Source: CAD feature listing. Evaluate the final solid. Frame: model axes, mm. A direction names the side the tool comes from. Round coordinates to 2 decimals unless told otherwise and drop trailing zeros. Order: outer loops, then holes, each group sorted by start corner. A loop starts at its lowest first (then second) coordinate and runs counter-clockwise, first axis right, second up. Notation, with made-up numbers: (-20.5, 6) - (-0.5, 6) arc R15 cw to (-0.5, 26) - close; hole circle Ø5 at (61.5, 60.5). An arc over 180 degrees is marked (long way). Use one line per item in the form item = value. Start each with the question number.
Q1. Cut plane B-B, the plane x = -17. Return the cut outline in (y, z) (3 decimals), and give its area (3 significant figures).
Q2. Set-up query: faces 5 (the cylindrical face through (-16.41, 1.97, 22.26)), 6 (the cylindrical face through (16.41, 1.97, 0.6)), 7 (the flat face through (-14, -1, 19.685)), 8 (the cylindrical face through (16.37, 1.97, 22.26)), 9 (the flat face through (-10.643, -1, 21)). Return all of +Z, -Z, +X, -X, +Y, -Y with unobstructed straight access to the full face (end or side cutting, diameter ignored); none if empty.
Q3. Pin query (flat end, axial travel): pin 1 Ø3.5 at (x, z) = (20.17, 11.43) entering from +Y; pin 2 Ø1.3 at (y, z) = (-1.5, 2) entering from +X; pin 3 Ø3 at (y, z) = (-1, 2) entering from -X. Return the tip coordinate at first contact, or that it passes through.
Q4. Cut plane C-C, the plane x = 0. Return the cut outline in (y, z), and give its area (3 significant figures).
Q5. Ray query, line 1 (X direction, y = 1.05, z = 11.43); line 2 (Y direction, x = 25.5, z = 11.75); line 3 (X direction, y = 3.75, z = 8.5). Return the intervals inside material, ascending. Write a range as [from, to].
Q6. Draft query along X for faces 1 (the cylindrical face through (-13.94, 2.95, 11.3)), 2 (the flat face through (10.643, -1, 2)), 3 (the cylindrical face through (-18.657, 1.288, 11.232)), 4 (the cylindrical face through (0.248, 13.815, 11.298)). Return one class per face: released by +X, released by -X, zero draft, split by the parting line, or undercut.
Q7. Cut plane A-A, the plane z = 11.43. Return the cut outline in (x, y), and give its area (3 significant figures).
from build123d import *

# Parameters (mm, degrees)
BOSS_EXTRUDE1_DEPTH      = 22.86
BOSS_EXTRUDE8_DEPTH      = 2.54
BOSS_EXTRUDE8_DEPTH_BACK = 2.54
SKETCH9_W                = 3.175
SKETCH9_H                = 22.86
BOSS_EXTRUDE9_DEPTH      = 2.54
BOSS_EXTRUDE9_DEPTH_BACK = 2.54
SKETCH10_W               = 3.175
SKETCH10_H               = 22.86
BOSS_EXTRUDE10_DEPTH     = 3.81
BOSS_EXTRUDE11_DEPTH     = 3.81
REVOLVE1_ANGLE           = 180
REVOLVE2_ANGLE           = 180
SKETCH22_W               = 16.51
SKETCH22_H               = 2.54
CUT_EXTRUDE1_DEPTH       = 3.81
SKETCH23_W               = 16.51
SKETCH23_H               = 2.54
CUT_EXTRUDE2_DEPTH       = 3.81
SKETCH24_R               = 1.524
CUT_EXTRUDE3_DEPTH       = 3.81
FILLET1_R                = 2


with BuildPart() as part:
    # Sketch1 → Boss-Extrude1 (new body)
    with BuildSketch(Plane.XY):
        with BuildLine():
            Line((-13.8176, 0), (-10.6426, 0))
            ThreePointArc((-10.6426, 0), (0, 10.6426), (10.6426, 0))
            Line((10.6426, 0), (13.8176, 0))
            ThreePointArc((13.8176, 0), (0, 13.8176), (-13.8176, 0))
        make_face()
    extrude(amount=BOSS_EXTRUDE1_DEPTH)

    # Sketch9 → Boss-Extrude8 (add, two sides: drawn at the far end of the back side and taken through both)
    with BuildSketch(Plane.XZ.offset(-BOSS_EXTRUDE8_DEPTH_BACK)):
        with Locations((-12.2301, 11.43)):
            Rectangle(SKETCH9_W, SKETCH9_H)
    extrude(amount=BOSS_EXTRUDE8_DEPTH + BOSS_EXTRUDE8_DEPTH_BACK)

    # Sketch10 → Boss-Extrude9 (add, two sides: drawn at the far end of the back side and taken through both)
    with BuildSketch(Plane.XZ.offset(-BOSS_EXTRUDE9_DEPTH_BACK)):
        with Locations((12.2301, 11.43)):
            Rectangle(SKETCH10_W, SKETCH10_H)
    extrude(amount=BOSS_EXTRUDE9_DEPTH + BOSS_EXTRUDE9_DEPTH_BACK)

    # Sketch11 → Boss-Extrude10 (add)
    with BuildSketch(Plane.ZY.offset(13.8176)):
        Polygon((22.86, 2.54), (0, 2.54), (0, 0), (0, -2.54), (3.175, -2.54), (3.175, 0), (19.685, 0), (19.685, -2.54), (22.86, -2.54), align=None)
    extrude(amount=BOSS_EXTRUDE10_DEPTH)

    # Sketch19 → Boss-Extrude11 (add)
    with BuildSketch(Plane(origin=(13.8176, 0, 0), x_dir=(0, 0, -1), z_dir=(1, 0, 0))):
        Polygon((-19.685, -2.54), (-19.685, 0), (-3.175, 0), (-3.175, -2.54), (0, -2.54), (0, 2.54), (-22.86, 2.54), (-22.86, -2.54), align=None)
    extrude(amount=BOSS_EXTRUDE11_DEPTH)

    # Sketch20 → Revolve1 (revolve)
    with BuildSketch(Plane.ZY.offset(17.6276)):
        Polygon((11.43, 2.54), (11.43, 0), (19.685, 0), (19.685, -2.54), (22.86, -2.54), (22.86, 2.54), align=None)
    revolve(axis=Axis((-17.6276, 2.54, 11.43), (0, -1, 0)), revolution_arc=REVOLVE1_ANGLE)

    # Sketch21 → Revolve2 (revolve)
    with BuildSketch(Plane(origin=(17.6276, 0, 0), x_dir=(0, 0, -1), z_dir=(1, 0, 0))):
        Polygon((-11.43, 2.54), (-11.43, 0), (-3.175, 0), (-3.175, -2.54), (0, -2.54), (0, 2.54), align=None)
    revolve(axis=Axis((17.6276, 2.54, 11.43), (0, -1, 0)), revolution_arc=REVOLVE2_ANGLE)

    # Sketch22 → Cut-Extrude1 (cut)
    with BuildSketch(Plane.ZY.offset(13.8176)):
        with Locations((11.43, -1.27)):
            Rectangle(SKETCH22_W, SKETCH22_H)
    extrude(amount=-CUT_EXTRUDE1_DEPTH, mode=Mode.SUBTRACT)

    # Sketch23 → Cut-Extrude2 (cut)
    with BuildSketch(Plane(origin=(13.8176, 0, 0), x_dir=(0, 0, -1), z_dir=(1, 0, 0))):
        with Locations((-11.43, -1.27)):
            Rectangle(SKETCH23_W, SKETCH23_H)
    extrude(amount=-CUT_EXTRUDE2_DEPTH, mode=Mode.SUBTRACT)

    # Sketch24 → Cut-Extrude3 (cut)
    with BuildSketch(Plane(origin=(0, 2.54, 0), x_dir=(1, 0, 0), z_dir=(0, 1, 0))):
        with Locations(Location((-20.1676, -11.43, 0), (0, 0, 270))):
            Circle(SKETCH24_R)
        with Locations(Location((20.1676, -11.43, 0), (0, 0, 270))):
            Circle(SKETCH24_R)
    extrude(amount=-CUT_EXTRUDE3_DEPTH, mode=Mode.SUBTRACT)

    # Fillet1
    fillet1_edges = [part.edges().sort_by_distance(p)[0] for p in [
        (-29.0576, 2.54, 11.43),
        (29.0576, 2.54, 11.43),
        (-15.604868947, 2.54, 0),
        (-15.604868947, 2.54, 22.86),
        (-13.582137894, 2.54, 11.43),
        (0, 13.8176, 0),
        (0, 13.8176, 22.86),
        (15.604868947, 2.54, 0),
        (15.604868947, 2.54, 22.86),
        (13.582137894, 2.54, 11.43),
    ]]
    fillet(fillet1_edges, radius=FILLET1_R)


solid = part.part
Completed:
q1.outline = (-2.54, 0) - (0.54, 0) arc R2 ccw to (2.54, 2) - (2.54, 20.86) arc R2 ccw to (0.54, 22.86) - (-2.54, 22.86) - (-2.54, 19.685) - (0, 19.685) - (0, 3.175) - (-2.54, 3.175) - close
q1.area = 72.5 mm2
q2.face_5 = +Z, -X, +Y
q2.face_6 = -Z, +X, +Y
q2.face_7 = -Y
q2.face_8 = +Z, +X, +Y
q2.face_9 = +Z, -Z, -Y
q3.pin_1 = 2.54
q3.pin_2 = 24.95
q3.pin_3 = -25.86
q4.outline = (10.64, 0) - (11.82, 0) arc R2 ccw to (13.82, 2) - (13.82, 20.86) arc R2 ccw to (11.82, 22.86) - (10.64, 22.86) - close
q4.area = 70.9 mm2
q5.line_1 = [-28.99, -21.69], [-18.64, -10.59], [10.59, 18.64], [21.69, 28.99]
q5.line_2 = [0, 2.54]
q5.line_3 = [-13.31, -9.96], [9.96, 13.31]
q6.face_1 = released by -X
q6.face_2 = undercut
q6.face_3 = undercut
q6.face_4 = split by the parting line
q7.outline = (-29.06, -2.54) - (-25.88, -2.54) - (-25.88, 0) - (-21.69, 0) - (-21.69, 2.54) - (-27.06, 2.54) arc R2 ccw to (-29.06, 0.54) - close; (-18.64, 0) - (-10.64, 0) arc R10.64 cw to (10.64, 0) - (18.64, 0) - (18.64, 2.54) - (15.15, 2.54) arc R2 cw to (13.24, 3.97) arc R13.82 ccw to (-13.24, 3.97) arc R2 cw to (-15.15, 2.54) - (-18.64, 2.54) - close; (21.69, 0) - (25.88, 0) - (25.88, -2.54) - (29.06, -2.54) - (29.06, 0.54) arc R2 ccw to (27.06, 2.54) - (21.69, 2.54) - close
q7.area = 200 mm2
